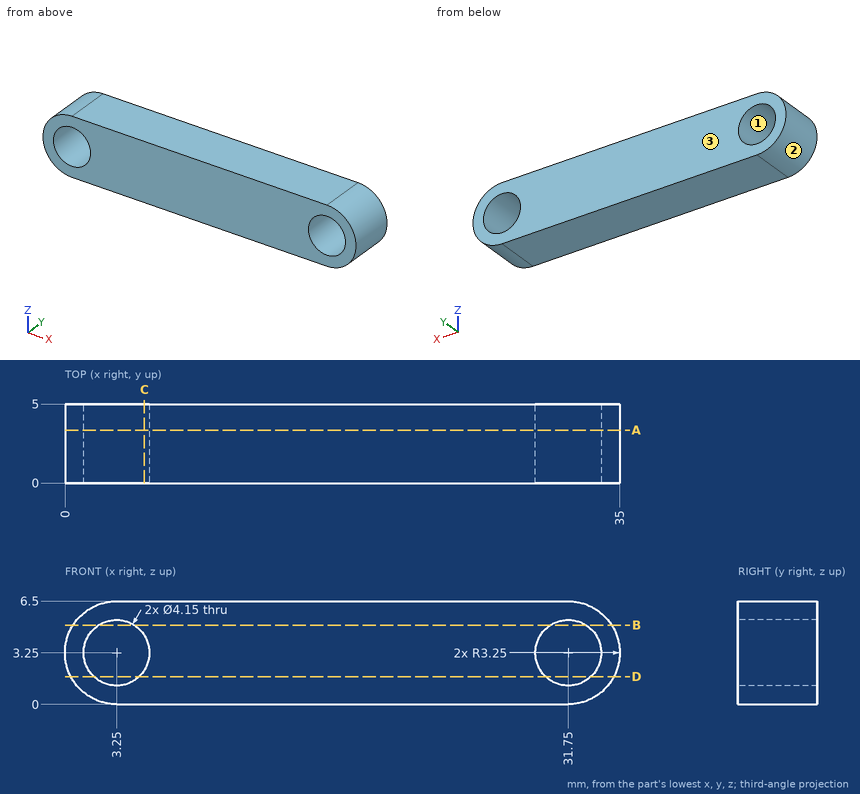
Drawing for the job (mm, zero at the part's lowest x, y, z). Round coordinates to 2 decimals unless told otherwise and drop trailing zeros. Write each loop counter-clockwise with the first axis right and the second up, starting at its lowest first coordinate (ties: lowest second). Pieces come first, ordered by that corner, then holes. Notation, with made-up numbers: (49, 5) - (108, 5) arc R19 cw to (108, 39) - close; hole circle Ø6 at (-15, 26). An arc over 180 degrees is marked (long way). Use CSV: the item, a comma, the result in double quotes.
(1) Pin check, flat tip, straight feed: P1, Ø3, axis at y = 3, z = 5.5, coming from the +X side. Stop position of the tip, or through.
Response:
P1,"x = 34.91"
(2) Band-saw the part on A-A (y = 3.35). Write the cut outline in (x, z) (3 decimals).
Response:
outline,"(3.25, 0) - (31.75, 0) arc R3.25 ccw to (31.75, 6.5) - (3.25, 6.5) arc R3.25 ccw to start; hole circle Ø4.15 at (3.25, 3.25); hole circle Ø4.15 at (31.75, 3.25)"
(3) Wall check: line 1 (Z direction, x = 3.25, y = 1.4) (3 decimals); line 2 (X direction, y = 0.85, z = 4.25); line 3 (X direction, y = 3.7, z = 3.5). Give the ranges that are in metal, low to high.
Response:
line 1,"0 to 1.175, 5.325 to 6.5"
line 2,"0.16 to 1.43, 5.07 to 29.93, 33.57 to 34.84"
line 3,"0.01 to 1.19, 5.31 to 29.69, 33.81 to 34.99"
(4) Band-saw the part on C-C (x = 5). Write the cut outline in (y, z).
Response:
outline,"(0, 0) - (5, 0) - (5, 2.14) - (0, 2.14) - close; (0, 4.36) - (5, 4.36) - (5, 6.5) - (0, 6.5) - close"
(5) Band-saw the part on B-B (z = 5). Write the cut outline in (x, y).
Response:
outline,"(0.51, 0) - (2.14, 0) - (2.14, 5) - (0.51, 5) - close; (4.36, 0) - (30.64, 0) - (30.64, 5) - (4.36, 5) - close; (32.86, 0) - (34.49, 0) - (34.49, 5) - (32.86, 5) - close"
(6) Band-saw the part on D-D (z = 1.75). Write the cut outline in (x, y).
Response:
outline,"(0.37, 0) - (1.82, 0) - (1.82, 5) - (0.37, 5) - close; (4.68, 0) - (30.32, 0) - (30.32, 5) - (4.68, 5) - close; (33.18, 0) - (34.63, 0) - (34.63, 5) - (33.18, 5) - close"
(7) Mould opens along Z. For the marked faces 1, 2 and 3 say: pulls with the +Z half, pulls with the -Z half, needs draft (parallel to the pull), parting line crosses it, or undercut.
Response:
face 1,"undercut"
face 2,"parting line crosses it"
face 3,"needs draft"
